```python
from build123d import *

# Parameters (mm, degrees)
SKETCH1_W           = 127.635
SKETCH1_H           = 127.635
BOSS_EXTRUDE1_DEPTH = 9.525
SKETCH12_R          = 83.82
BOSS_EXTRUDE2_DEPTH = 9.525
SKETCH13_R          = 104.928492752
SKETCH13_R_2        = 83.82
CUT_EXTRUDE4_DEPTH  = 9.525
SKETCH5_R           = 46.355
CUT_EXTRUDE1_DEPTH  = 9.525
SKETCH11_R          = 1.4351
CUT_EXTRUDE3_DEPTH  = 10.525
CIRPATTERN1_COUNT   = 12


with BuildPart() as part:
    # Sketch1 → Boss-Extrude1 (new body)
    with BuildSketch(Plane(origin=(0, 0, 0), x_dir=(1, 0, 0), z_dir=(0, 1, 0))):
        with Locations((63.8175, 63.8175)):
            Rectangle(SKETCH1_W, SKETCH1_H)
    extrude(amount=BOSS_EXTRUDE1_DEPTH)

    # Sketch12 → Boss-Extrude2 (add)
    with BuildSketch(Plane.XZ):
        with Locations((63.8175, -63.8175)):
            Circle(SKETCH12_R)
    extrude(amount=-BOSS_EXTRUDE2_DEPTH)

    # Sketch13 → Cut-Extrude4 (cut)
    with BuildSketch(Plane(origin=(0, 0, 0), x_dir=(-1, 0, 0), z_dir=(0, -1, 0))):
        with Locations((-63.8175, 63.8175)):
            Circle(SKETCH13_R)
        with Locations((-63.8175, 63.8175)):
            Circle(SKETCH13_R_2, mode=Mode.SUBTRACT)
    extrude(amount=-CUT_EXTRUDE4_DEPTH, mode=Mode.SUBTRACT)

    # Sketch5 → Cut-Extrude1 (cut)
    with BuildSketch(Plane(origin=(0, 9.525, 0), x_dir=(1, 0, 0), z_dir=(0, 1, 0))):
        with Locations((63.8175, 63.8175)):
            Circle(SKETCH5_R)
    extrude(amount=-CUT_EXTRUDE1_DEPTH, mode=Mode.SUBTRACT)

    # Sketch11 → Cut-Extrude3 (cut, through all)
    with BuildSketch(Plane(origin=(0, 9.525, 0), x_dir=(1, 0, 0), z_dir=(0, 1, 0))):
        with Locations((63.8175, 115.443)):
            Circle(SKETCH11_R)
    cut_extrude3 = extrude(amount=-CUT_EXTRUDE3_DEPTH, mode=Mode.SUBTRACT)

    # CirPattern1: Cut-Extrude3 ×12 about axis
    cirpattern1_axis = Axis((63.8175, 0, -63.8175), (0, 1, 0))
    for i in range(1, CIRPATTERN1_COUNT):
        add(cut_extrude3.rotate(cirpattern1_axis, i * 360 / CIRPATTERN1_COUNT), mode=Mode.SUBTRACT)


solid = part.part
```
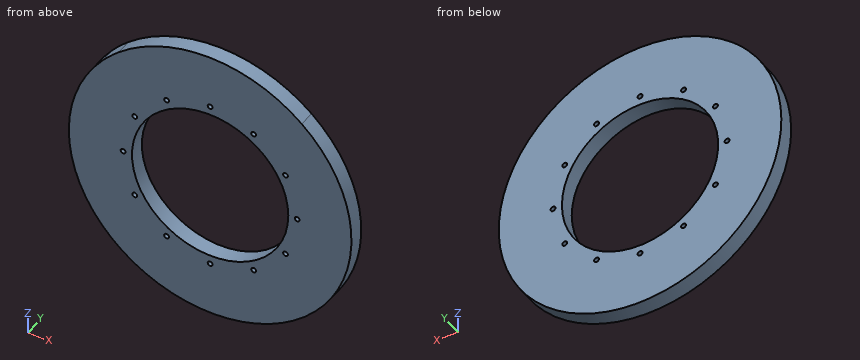
Build history of the part. All positions in model axes, mm. Round coordinates to 2 decimals unless told otherwise and drop trailing zeros. Write each loop counter-clockwise with the first axis right and the second up, starting at its lowest first coordinate (ties: lowest second). Pieces come first, ordered by that corner, then holes.
1) Band-saw the part on B-B, the plane z = -102.5. List the corners of the cut face in (x, y) (3 decimals), and give its area (3 significant figures).
2) Drill centre lines: probe 1 along X at (y, z) = (9, -89.5); probe 2 along X at (y, z) = (5, -99); probe 3 along Z at (x, y) = (99, 2.25). Where is each one in solid material? Low to high.
3) Band-saw the part on A-A, the plane x = 99.5. List the corners of the cut face in (y, z) (3 decimals).
4) Band-saw the part on D-D, the plane x = 123.5. List the corners of the cut face in (y, z) (3 decimals), and give its area (3 significant figures).
5) Band-saw the part on C-C, the plane y = 1.5. Give the number of separate pieces and of enclosed holes in the cut face, and give its area (3 significant figures).
6) Pin check, flat tips, straight feed: pin 1 (1.5 mm diameter, centred on y = 4, z = -52.5, fed in from +X); pin 2 (1 mm diameter, centred on x = 93, y = 8, fed in from -Z); pin 3 (3 mm diameter, centred on y = 4, z = -100.5, fed in from +X); pin 4 (1.7 mm diameter, centred on x = 115.44, z = -63.82, fed in from +Y). Stop position of each tip, or through.
Ans:
1. outline: (-10.543, 0) - (38.274, 0) - (38.274, 9.525) - (-10.543, 9.525) - close; (89.361, 0) - (138.178, 0) - (138.178, 9.525) - (89.361, 9.525) - close
1. area: 930 mm2
2. probe 1: x = -15.97 to 17.68, 20.54 to 25.23, 102.41 to 107.1, 109.96 to 143.61
2. probe 2: x = -12.26 to 33.64, 94 to 139.9
2. probe 3: z = -139.9 to -94, -33.64 to 12.26
3. outline: (0, -139.663) - (9.525, -139.663) - (9.525, -93.407) - (0, -93.407) - close; (0, -34.228) - (9.525, -34.228) - (9.525, 12.028) - (0, 12.028) - close
4. outline: (0, -122.671) - (9.525, -122.671) - (9.525, -4.964) - (0, -4.964) - close
4. area: 1,120 mm2
5. separate pieces: 1
5. enclosed holes: 13
5. area: 15,200 mm2
6. pin 1: stops at x = 146.97
6. pin 2: stops at z = -142.58
6. pin 3: stops at x = 139.9
6. pin 4: passes through
